Read the model definition and answer for the solid it produces. Units are mm, in the model's axes. Face numbers are marked on the shaded views. A direction names the side the tool comes from. Give positions to 0.01 mm unless a question says otherwise; leave off trailing zeros. Loops run counter-clockwise (first coordinate to the right, second up) from the corner with the lowest first, then second, coordinate; pieces in that order, holes last. Notation, with made-up numbers: (66.25, -13.75) -> (108.25, -13.75) arc R35 cw to (108.25, 18.25) -> close; hole circle Ø4 at (-17, -4). An arc over 180 degrees is marked (long way). Return JSON: item names as keys, results as strings. Group by question number.
from build123d import *

# Parameters (mm, degrees)
SKETCH_2_R      = 1.6
EXTRUDE_1_DEPTH = 15
FILLET_1_R      = 3
SKETCH_3_W      = 45
SKETCH_3_H      = 12
SKETCH_3_R      = 1.55
EXTRUDE_2_DEPTH = 15
FILLET_2_R      = 3


with BuildPart() as part:
    # 草图2 → 凸台-拉伸1 (new body)
    with BuildSketch(Plane.XY):
        with BuildLine():
            Line((110.262395693, 45.951905284), (110.262395693, 72.951905284))
            Line((110.262395693, 72.951905284), (75.937822174, 13.5))
            ThreePointArc((75.937822174, 13.5), (74.839745962, 12.401923789), (73.339745962, 12))
            Line((73.339745962, 12), (0, 12))
            Line((0, 12), (0, 0))
            Line((0, 0), (80.267949192, 0))
            ThreePointArc((80.267949192, 0), (81.767949192, 0.401923789), (82.866025404, 1.5))
            Line((82.866025404, 1.5), (107.664319482, 44.451905284))
            ThreePointArc((107.664319482, 44.451905284), (108.762395693, 45.549981495), (110.262395693, 45.951905284))
        make_face()
        with Locations((99.292740578, 41.951905284)):
            Circle(SKETCH_2_R, mode=Mode.SUBTRACT)
        with Locations((89.292740578, 24.631397208)):
            Circle(SKETCH_2_R, mode=Mode.SUBTRACT)
        with Locations((67, 6)):
            Circle(SKETCH_2_R, mode=Mode.SUBTRACT)
        with Locations((37, 6)):
            Circle(SKETCH_2_R, mode=Mode.SUBTRACT)
        with Locations((7, 6)):
            Circle(SKETCH_2_R, mode=Mode.SUBTRACT)
    extrude(amount=EXTRUDE_1_DEPTH)

    # 圆角1
    fillet_1_edges = [part.edges().sort_by_distance(p)[0] for p in [
        (0, 0, 7.5),
        (0, 12, 7.5),
        (110.262395693, 72.951905284, 7.5),
        (110.262395693, 45.951905284, 7.5),
    ]]
    fillet(fillet_1_edges, radius=FILLET_1_R)

    # 草图3 → 凸台-拉伸2 (add)
    with BuildSketch(Plane.XY.offset(15)):
        with Locations((-19.5, 6)):
            Rectangle(SKETCH_3_W, SKETCH_3_H)
        with Locations((-23, 6)):
            Circle(SKETCH_3_R, mode=Mode.SUBTRACT)
    extrude(amount=-EXTRUDE_2_DEPTH)

    # 圆角2
    fillet_2_edges = [part.edges().sort_by_distance(p)[0] for p in [
        (-42, 0, 7.5),
        (-42, 12, 7.5),
    ]]
    fillet(fillet_2_edges, radius=FILLET_2_R)


solid = part.part
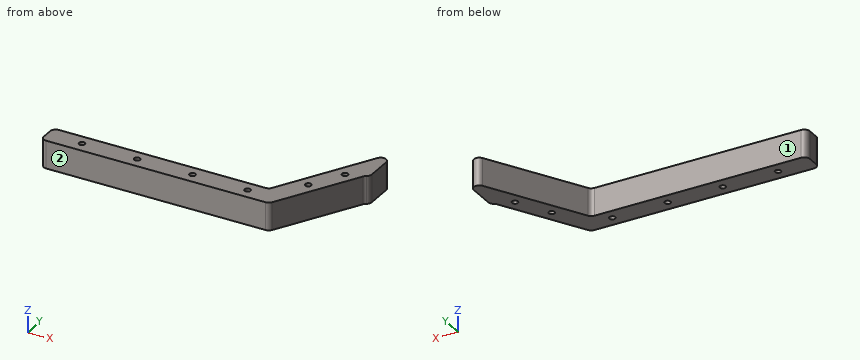
1. Section B-B on z = 4.5 is taken. Determine the outline of the cut face in (x, y), then the cut area to 3 significant figures.
2. Flat-ended cylindrical pins translate along their axes: pin 1 Ø3.5 at (x, y) = (89.29, 24.63) entering from +Z; pin 2 Ø3 at (y, z) = (50.5, 4.5) entering from -X; pin 3 Ø4.5 at (x, z) = (29.5, 9.5) entering from +Y; pin 4 Ø6 at (y, z) = (20, 4.5) entering from -X. Find the tip coordinate at first contact, or state that the pin passes through.
3. Section D-D on x = -23 is taken. Determine the outline of the cut face in (y, z), then the cut area to 4 significant figures.
4. Section C-C on y = 6 is taken. Determine the outline of the cut face in (x, z).
5. Which of the six approach directions +Z, -Z, +X, -X, +Y, -Y give full straight-line access (tool end or side, diameter ignored) to the marked faces 1 and 2?
6. Straight lines are drawn through the part: line 1 (Y direction, x = -23, z = 9.25); line 2 (Y direction, x = 37, z = 10.25); line 3 (Y direction, x = 62.5, z = 14). For each, find the intervals that lie inside material, in ascending order. Write a range as from..to.
7. Section A-A on x = 7 is taken. Determine the outline of the cut face in (y, z).
Completed:
{
 "1": {"outline": "(-42, 3) arc R3 ccw to (-39, 0) -> (80.27, 0) arc R3 ccw to (82.87, 1.5) -> (107.66, 44.45) arc R3 cw to (108.76, 45.55) arc R3 ccw to (110.26, 48.15) -> (110.26, 61.76) arc R3 ccw to (104.66, 63.26) -> (75.94, 13.5) arc R3 cw to (73.34, 12) -> (-39, 12) arc R3 ccw to (-42, 9) -> close; hole circle Ø3.1 at (-23, 6); hole circle Ø3.2 at (7, 6); hole circle Ø3.2 at (37, 6); hole circle Ø3.2 at (67, 6); hole circle Ø3.2 at (89.29, 24.63); hole circle Ø3.2 at (99.29, 41.95)", "area": "2,140 mm²"},
 "2": {"pin 1": "stops at z = 15", "pin 2": "stops at x = 96.43", "pin 3": "stops at y = 12", "pin 4": "stops at x = 77.96"},
 "3": {"outline": "(0, 0) -> (4.45, 0) -> (4.45, 15) -> (0, 15) -> close; (7.55, 0) -> (12, 0) -> (12, 15) -> (7.55, 15) -> close", "area": "133.5 mm²"},
 "4": {"outline": "(-42, 0) -> (-24.55, 0) -> (-24.55, 15) -> (-42, 15) -> close; (-21.45, 0) -> (5.4, 0) -> (5.4, 15) -> (-21.45, 15) -> close; (8.6, 0) -> (35.4, 0) -> (35.4, 15) -> (8.6, 15) -> close; (38.6, 0) -> (65.4, 0) -> (65.4, 15) -> (38.6, 15) -> close; (68.6, 0) -> (85.46, 0) -> (85.46, 15) -> (68.6, 15) -> close"},
 "5": {"face 1": "+Z, -Z, -X, +Y", "face 2": "+Z, -Z, +X, -X, -Y"},
 "6": {"line 1": "y = 0..4.45, 7.55..12", "line 2": "y = 0..4.4, 7.6..12", "line 3": "y = 0..12"},
 "7": {"outline": "(0, 0) -> (4.4, 0) -> (4.4, 15) -> (0, 15) -> close; (7.6, 0) -> (12, 0) -> (12, 15) -> (7.6, 15) -> close"}
}
